Could you check a few things on this model? Use its own coordinates, in mm. Face numbers are marked on the shaded views. A direction names the side the tool comes from. Coordinates: 2 decimals unless noted, no trailing zeros. Write each loop counter-clockwise with the first axis right and the second up, starting at its lowest first coordinate (ties: lowest second). Pieces come first, ordered by that corner, then holes. Notation, with made-up numbers: (27.25, 11) - (67.25, 11) arc R21 cw to (67.25, 35) - close; hole circle Ø10 at (24.5, -40). An arc over 180 degrees is marked (long way). Answer as a JSON object with one key per item and string values. Group by question number.
1) If we section it at C-C (y = -7): Write out the boundary of the cut face in (x, z) (3 decimals), plus the area to 3 significant figures.
2) On a 3-axis mill with a long thin cutter (end or side, diameter ignored), from which of +Z, -Z, +X, -X, +Y, -Y can I reach the whole of each face in a straight line? I mean the marked faces 5, 6 and 7. Say none if no direction works.
3) Please list where these lines run through material, in increasing order: line 1 along X through (y, z) = (-4, 6.5); line 2 along Y through (x, z) = (19, -4); line 3 along X through (y, z) = (0.75, -13.25).
4) If we section it at B-B (x = 1): Write out the boundary of the cut face in (y, z) (3 decimals).
5) If we section it at D-D (y = -3): Write out the boundary of the cut face in (x, z) (3 decimals), plus the area to 3 significant figures.
6) We'd pull the mould along X, two halves only. Please class the marked faces 1, 2, 3 and 4: released by +X, released by -X, zero draft, split by the parting line, or undercut.
7) If we section it at A-A (z = 5): Write out the boundary of the cut face in (x, y), plus the area to 3 significant figures.
8) Will these pins go through, and if not, where does the flat tip stop? pin 1 Ø8 at (y, z) = (-13, -8) entering from -X; pin 2 Ø3 at (x, z) = (-1, -13) entering from -Y; pin 3 Ø5 at (x, y) = (-10, -12.5) entering from -Z; pin 4 Ø3.5 at (x, y) = (0, -5) entering from +Z (3 decimals).
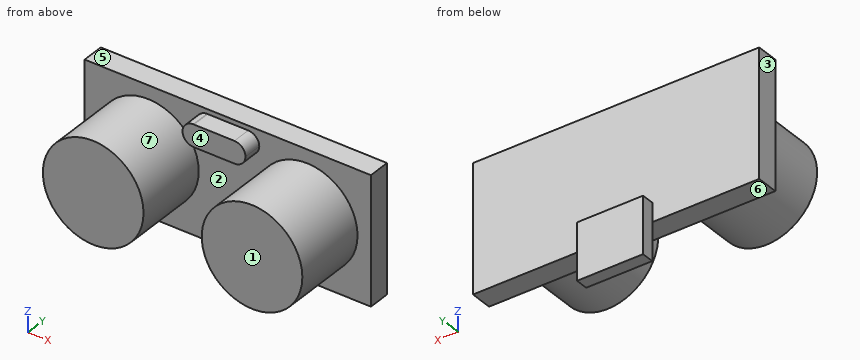
```python
from build123d import *

# Parameters (mm, degrees)
F0_R     = 8
F0_W     = 10.5
F0_H     = 3
F1_DEPTH = 3.5
F2_DEPTH = 15.5
F3_DEPTH = 6.5
F0_H_2   = 6
F4_DEPTH = 2


with BuildPart() as f1:
    # F0 (on Front) → F1 (new body)
    with BuildSketch(Plane.XZ):
        Polygon((22.75, 10.125), (-22.75, 10.125), (-22.75, -10.125), (-5.75, -10.125), (-5.75, -7.125), (4.75, -7.125), (4.75, -10.125), (22.75, -10.125), align=None)
        with Locations((-12.625, 0)):
            Circle(F0_R, mode=Mode.SUBTRACT)
        with Locations((12.625, 0)):
            Circle(F0_R, mode=Mode.SUBTRACT)
        with BuildLine():
            ThreePointArc((-3.25, 5.8816159739), (-4.9996694778, 7.5976054108), (-3.3180082792, 9.38029401))
            ThreePointArc((-3.3180082792, 9.38029401), (-3.2503522375, 9.3816159385), (-3.1826956692, 9.3803212456))
            Line((-3.1826956692, 9.3803212456), (3.2496477625, 9.3816159385))
            ThreePointArc((3.2496477625, 9.3816159385), (4.487312326, 8.8691773695), (5, 7.6316159739))
            ThreePointArc((5, 7.6316159739), (4.4874368671, 6.3941791069), (3.25, 5.8816159739))
            Line((3.25, 5.8816159739), (-3.25, 5.8816159739))
        make_face(mode=Mode.SUBTRACT)
        with Locations((-0.5, -8.625)):
            Rectangle(F0_W, F0_H)
        with Locations((-12.625, 0)):
            Circle(F0_R)
        with Locations((12.625, 0)):
            Circle(F0_R)
        with BuildLine():
            ThreePointArc((-3.1826956692, 9.3803212456), (-3.2503522375, 9.3816159385), (-3.3180082792, 9.38029401))
            Line((-3.3180082792, 9.38029401), (-3.1826956692, 9.3803212456))
        make_face()
    extrude(amount=F1_DEPTH)

    # F0 (on Front) → F2 (join)
    with BuildSketch(Plane.XZ):
        with Locations((-12.625, 0)):
            Circle(F0_R)
        with Locations((12.625, 0)):
            Circle(F0_R)
    extrude(amount=F2_DEPTH)

    # F0 (on Front) → F3 (join)
    with BuildSketch(Plane.XZ):
        with BuildLine():
            Line((3.2496477625, 9.3816159385), (-3.1826956692, 9.3803212456))
            ThreePointArc((-3.1826956692, 9.3803212456), (-1.988991955, 8.8450238652), (-1.5, 7.6316159739))
            Line((-1.5, 7.6316159739), (1.5, 7.6316159739))
            ThreePointArc((1.5, 7.6316159739), (2.0124386044, 8.8689283), (3.2496477625, 9.3816159385))
        make_face()
        with BuildLine():
            ThreePointArc((-1.5, 7.6316159739), (-2.0125631329, 6.3941791069), (-3.25, 5.8816159739))
            Line((-3.25, 5.8816159739), (3.25, 5.8816159739))
            ThreePointArc((3.25, 5.8816159739), (2.0125631329, 6.3941791069), (1.5, 7.6316159739))
            Line((1.5, 7.6316159739), (-1.5, 7.6316159739))
        make_face()
        with BuildLine():
            Line((-3.1826956692, 9.3803212456), (-3.3180082792, 9.38029401))
            ThreePointArc((-3.3180082792, 9.38029401), (-4.9996694778, 7.5976054108), (-3.25, 5.8816159739))
            ThreePointArc((-3.25, 5.8816159739), (-2.0125631329, 6.3941791069), (-1.5, 7.6316159739))
            ThreePointArc((-1.5, 7.6316159739), (-1.988991955, 8.8450238652), (-3.1826956692, 9.3803212456))
        make_face()
        with BuildLine():
            ThreePointArc((1.5, 7.6316159739), (2.0125631329, 6.3941791069), (3.25, 5.8816159739))
            ThreePointArc((3.25, 5.8816159739), (4.4874368671, 6.3941791069), (5, 7.6316159739))
            ThreePointArc((5, 7.6316159739), (4.487312326, 8.8691773695), (3.2496477625, 9.3816159385))
            ThreePointArc((3.2496477625, 9.3816159385), (2.0124386044, 8.8689283), (1.5, 7.6316159739))
        make_face()
    extrude(amount=F3_DEPTH)

    # F0 (on Front) → F4 (join)
    with BuildSketch(Plane.XZ):
        with Locations((-0.5, -8.625)):
            Rectangle(F0_W, F0_H)
        with Locations((-0.5, -13.125)):
            Rectangle(F0_W, F0_H_2)
    extrude(amount=-F4_DEPTH)


solid = f1.part
```
Here are the results:
{
 "1": {"outline": "circle Ø16 at (-12.625, 0); circle Ø16 at (12.625, 0)", "area": "402 mm²"},
 "2": {"face 5": "+Z, +X, -X, +Y, -Y", "face 6": "-Z, +X, -X, -Y", "face 7": "-Y"},
 "3": {"line 1": "x = -17.29 to -7.96, -4.58 to 4.58, 7.96 to 17.29", "line 2": "y = -15.5 to 0", "line 3": "x = -5.75 to 4.75"},
 "4": {"outline": "(-6.5, 5.882) - (-3.5, 5.882) - (-3.5, -10.125) - (0, -10.125) - (0, -16.125) - (2, -16.125) - (2, -7.125) - (0, -7.125) - (0, 10.125) - (-3.5, 10.125) - (-3.5, 9.381) - (-6.5, 9.381) - close"},
 "5": {"outline": "(-22.75, -10.125) - (22.75, -10.125) - (22.75, 10.125) - (-22.75, 10.125) - close", "area": "921 mm²"},
 "6": {"face 1": "zero draft", "face 2": "undercut", "face 3": "released by -X", "face 4": "undercut"},
 "7": {"outline": "(-22.75, -3.5) - (-18.87, -3.5) - (-18.87, -15.5) - (-6.38, -15.5) - (-6.38, -3.5) - (6.38, -3.5) - (6.38, -15.5) - (18.87, -15.5) - (18.87, -3.5) - (22.75, -3.5) - (22.75, 0) - (-22.75, 0) - close", "area": "459 mm²"},
 "8": {"pin 1": "stops at x = -19.55", "pin 2": "stops at y = 0", "pin 3": "stops at z = -8", "pin 4": "stops at z = 10.125"}
}
